Design review of the part shown in the three views and the two pictorial views. Dimensions are in mm from the part's minimum x, y and z. Round coordinates to 2 decimals unless told otherwise and drop trailing zeros. Order: outer loops, then holes, each group sorted by start corner. A loop starts at its lowest first (then second) coordinate and runs counter-clockwise, first axis right, second up.
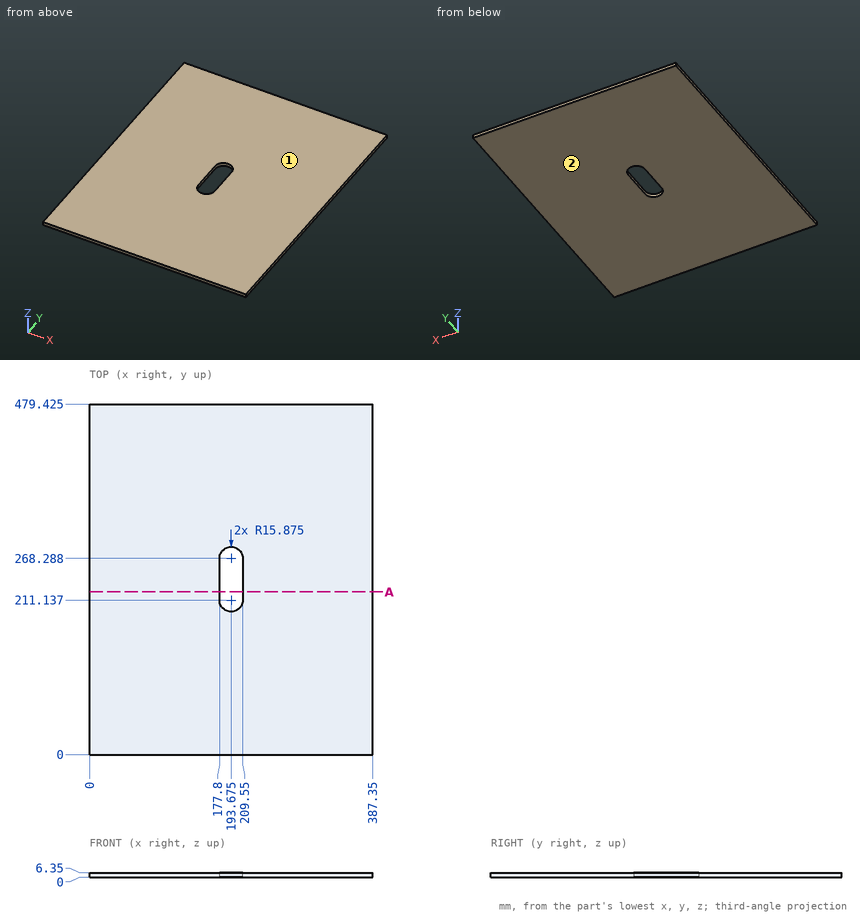
1) To check wall thickness, follow line 1 along X through (y, z) = (256.5, 3); line 2 along Y through (x, z) = (193, 4.75) (1 decimal); line 3 along Y through (x, z) = (182, 1) (1 decimal). State the ranges of each line that lie inside material, in increasing order.
Results:
line 1: x = 0 to 177.8, 209.55 to 387.35
line 2: y = 0 to 195.3, 284.1 to 479.4
line 3: y = 0 to 200.4, 279 to 479.4
2) The part is to be moulded in two halves that separate along Z. For the marked faces 1 and 2, say which applies: released by +Z, released by -Z, zero draft, split by the parting line, or undercut.
Results:
face 1: released by +Z
face 2: released by -Z
3) Clearance check with a flat-ended pin moving along its axis: P1, Ø1, axis at x = 119.5, z = 4, coming from the -Y side. State where the tip first meets the part, or that it passes through.
Results:
P1: stops at y = 0
4) Take a section at A-A on y = 222.5. Give the boundary of the cut face in (x, z), plus the area to 3 significant figures.
Results:
outline: (0, 0) - (177.8, 0) - (177.8, 6.35) - (0, 6.35) - close; (209.55, 0) - (387.35, 0) - (387.35, 6.35) - (209.55, 6.35) - close
area: 2,260 mm2
